For this review, take the finished solid that the model builds, in its own axes (mm). Face numbers are marked on the shaded views. A direction names the side the tool comes from. Round coordinates to 2 decimals unless told otherwise and drop trailing zeros. Loops run counter-clockwise (first coordinate to the right, second up) from the corner with the lowest first, then second, coordinate; pieces in that order, holes last. Notation, with made-up numbers: M 66,29.25 L 89,29.25 A22 cw 89,57.25 Z; hole C 41.25,78.25 d2. An arc over 180 degrees is marked long. Write item = value, one per line. Start each with the question number.
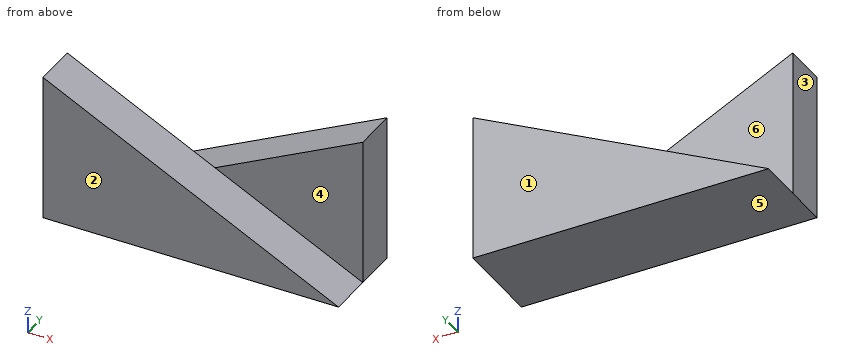
```python
from build123d import *

# Parameters (mm, degrees)
F1_DEPTH = 19.05
F2_DEPTH = 19.05


with BuildPart() as f1:
    # F0 (on Front) → F1 (new body)
    with BuildSketch(Plane.XZ):
        Polygon((-63.5, 31.75), (-63.5, -31.75), (0, 0), align=None)
        Polygon((-63.5, -31.75), (63.5, -31.75), (0, 0), align=None)
    extrude(amount=F1_DEPTH)

    # F0 (on Front) → F2 (join)
    with BuildSketch(Plane.XZ):
        Polygon((0, 0), (63.5, -31.75), (63.5, 31.75), align=None)
        Polygon((-63.5, -31.75), (63.5, -31.75), (0, 0), align=None)
    extrude(amount=-F2_DEPTH)


solid = f1.part
```
(1) Wall thickness on L1, parallel to Y at x = -54, z = -16; L2, parallel to Y at x = 58, z = 25; L3, parallel to Z at x = -1.5, y = -9: over which ranges is each line inside the solid? List them lowest first.
(2) Add section B-B on z = -19.5. Write out the cut boundary in (x, y), and give its area (3 significant figures).
(3) Add section D-D on y = -9. Write out the cut boundary in (x, z).
(4) Draft analysis for pull direction Y (two halves, no side actions). For the marked faces 1, 2 and 3, state which applies: +Y half, -Y half, draft (parallel to the pull), parting line (faces both ways), or undercut.
(5) Add section A-A on z = 12.5. Write out the cut boundary in (x, y).
(6) Tool access review of the marked faces 4, 5 and 6: name each direction out of +Z, -Z, +X, -X, +Y, -Y from which nothing blocks a thin tool from reaching the whole face with its end or side.
(7) For pin 1 Ø1 at (x, z) = (-34.5, -5.5) entering from +Y; pin 2 Ø5 at (x, y) = (34, 14) entering from +Z; pin 3 Ø4 at (x, y) = (-24.5, 7) entering from +Z, all flat-tipped, find the tip position at first contact; note any pin that passes through.
(8) Add section C-C on x = 38. Write out the cut boundary in (y, z), and give its area (3 significant figures).
Answer sheet:
q1.L1 = -19.05 to 0
q1.L2 = 0 to 19.05
q1.L3 = -31.75 to 0.75
q2.outline = M -63.5,-19.05 L 39,-19.05 L 39,0 L 63.5,0 L 63.5,19.05 L -39,19.05 L -39,0 L -63.5,0 Z
q2.area = 3,910 mm²
q3.outline = M -63.5,-31.75 L 63.5,-31.75 L -63.5,31.75 Z
q4.face_1 = +Y half
q4.face_2 = -Y half
q4.face_3 = draft
q5.outline = M -63.5,-19.05 L -25,-19.05 L -25,0 L -63.5,0 Z; M 25,0 L 63.5,0 L 63.5,19.05 L 25,19.05 Z
q6.face_4 = +Z, +X, -Y
q6.face_5 = -Z, +X, -X, +Y, -Y
q6.face_6 = +Z, -X, +Y
q7.pin_1 = 0
q7.pin_2 = 18.25
q7.pin_3 = -11.25
q8.outline = M -19.05,-31.75 L 19.05,-31.75 L 19.05,19 L 0,19 L 0,-19 L -19.05,-19 Z
q8.area = 1,210 mm²
